```python
from build123d import *

# Parameters (mm, degrees)
SKETCH1_W                      = 247
SKETCH1_H                      = 127
BOSS_EXTRUDE1_DEPTH            = 63.5
M3X0_5_TAPPED_HOLE1_AT_2_COUNT = 2
M3X0_5_TAPPED_HOLE1_AT_2_PITCH = 20
M3X0_5_TAPPED_HOLE1_AT_3_COUNT = 2
M3X0_5_TAPPED_HOLE1_AT_3_PITCH = 220.907220344
M3X0_5_TAPPED_HOLE1_AT_4_COUNT = 2
M3X0_5_TAPPED_HOLE1_AT_4_PITCH = 220
SKETCH4_W                      = 19.05
SKETCH4_H                      = 6.35
BOSS_EXTRUDE2_DEPTH            = 5
SKETCH5_W                      = 1.5875
SKETCH5_H                      = 6.35
BOSS_EXTRUDE3_DEPTH            = 5


with BuildPart() as part:
    # Sketch1 → Boss-Extrude1 (new body)
    with BuildSketch(Plane(origin=(0, 0, 0), x_dir=(1, 0, 0), z_dir=(0, 1, 0))):
        Rectangle(SKETCH1_W, SKETCH1_H)
    extrude(amount=BOSS_EXTRUDE1_DEPTH)

    # Sketch3 → M3x0.5 Tapped Hole1 (revolve, cut)
    with BuildSketch(Plane(origin=(-112.5, 33.5, 63.5), x_dir=(0, -1, 0), z_dir=(1, 0, 0))):
        Polygon((0, 0), (0, 4.751075774), (1.25, 4), (1.25, 0), align=None)
    m3x0_5_tapped_hole1 = revolve(axis=Axis((-112.5, 33.5, 69.85), (0, 0, -1)), mode=Mode.SUBTRACT)

    # M3x0.5 Tapped Hole1 at 2: M3x0.5 Tapped Hole1 ×2
    with Locations(*[(0, -i * M3X0_5_TAPPED_HOLE1_AT_2_PITCH, 0) for i in range(1, M3X0_5_TAPPED_HOLE1_AT_2_COUNT)]):
        add(m3x0_5_tapped_hole1, mode=Mode.SUBTRACT)

    # M3x0.5 Tapped Hole1 at 3: M3x0.5 Tapped Hole1 ×2
    with Locations(*[Vector(0.9958932064677039, -0.09053574604251853, 0) * (i * M3X0_5_TAPPED_HOLE1_AT_3_PITCH) for i in range(1, M3X0_5_TAPPED_HOLE1_AT_3_COUNT)]):
        add(m3x0_5_tapped_hole1, mode=Mode.SUBTRACT)

    # M3x0.5 Tapped Hole1 at 4: M3x0.5 Tapped Hole1 ×2
    with Locations(*[(i * M3X0_5_TAPPED_HOLE1_AT_4_PITCH, 0, 0) for i in range(1, M3X0_5_TAPPED_HOLE1_AT_4_COUNT)]):
        add(m3x0_5_tapped_hole1, mode=Mode.SUBTRACT)

    # Mirror1: M3x0.5 Tapped Hole1 across plane
    add(m3x0_5_tapped_hole1.mirror(Plane.XY), mode=Mode.SUBTRACT)

    # Mirror1 copy 1 sketch → Mirror1 copy 1 (revolve, cut)
    with BuildSketch(Plane(origin=(-112.5, 13.5, -63.5), x_dir=(0, -1, 0), z_dir=(1, 0, 0))):
        Polygon((0, 0), (0, -4.751075774), (1.25, -4), (1.25, 0), align=None)
    revolve(axis=Axis((-112.5, 13.5, -69.85), (0, 0, -1)), mode=Mode.SUBTRACT)

    # Mirror1 copy 2 sketch → Mirror1 copy 2 (revolve, cut)
    with BuildSketch(Plane(origin=(107.5, 13.5, -63.5), x_dir=(0, -1, 0), z_dir=(1, 0, 0))):
        Polygon((0, 0), (0, -4.751075774), (1.25, -4), (1.25, 0), align=None)
    revolve(axis=Axis((107.5, 13.5, -69.85), (0, 0, -1)), mode=Mode.SUBTRACT)

    # Mirror1 copy 3 sketch → Mirror1 copy 3 (revolve, cut)
    with BuildSketch(Plane(origin=(107.5, 33.5, -63.5), x_dir=(0, -1, 0), z_dir=(1, 0, 0))):
        Polygon((0, 0), (0, -4.751075774), (1.25, -4), (1.25, 0), align=None)
    revolve(axis=Axis((107.5, 33.5, -69.85), (0, 0, -1)), mode=Mode.SUBTRACT)

    # Sketch4 → Boss-Extrude2 (add)
    with BuildSketch(Plane.ZY.offset(123.5)):
        with Locations((38.975, 15.175)):
            Rectangle(SKETCH4_W, SKETCH4_H)
    extrude(amount=BOSS_EXTRUDE2_DEPTH)

    # Sketch5 → Boss-Extrude3 (add)
    with BuildSketch(Plane.ZY.offset(128.5)):
        with Locations((30.24375, 15.175)):
            Rectangle(SKETCH5_W, SKETCH5_H)
        with Locations((36.064583333, 15.175)):
            Rectangle(SKETCH5_W, SKETCH5_H)
        with Locations((47.70625, 15.175)):
            Rectangle(SKETCH5_W, SKETCH5_H)
        with Locations((41.885416667, 15.175)):
            Rectangle(SKETCH5_W, SKETCH5_H)
    extrude(amount=BOSS_EXTRUDE3_DEPTH)


solid = part.part
```
Build history of the part. All positions in model axes, mm. A direction names the side the tool comes from. Coordinates: 2 decimals unless noted, no trailing zeros. Order: outer loops, then holes, each group sorted by start corner. A loop starts at its lowest first (then second) coordinate and runs counter-clockwise, first axis right, second up.
Item 1: Tool access for faces 4 (the flat face through (-127, 18.35, 39)), 5 (the flat face through (-127, 12, 39)), 6 (the flat face through (-131, 15, 42.679)): list every direction of +Z, -Z, +X, -X, +Y, -Y with a clear straight run to the whole face (end or side of a thin tool).
Filled in:
face 4: +Z, -Z, -X, +Y
face 5: +Z, -Z, -X, -Y
face 6: -X, +Y, -Y
Item 2: Saw through at A-A on y = 57.5. List the corners of the cut face in (x, z), then the cut area to 3 significant figures.
Filled in:
outline: (-123.5, -63.5) - (123.5, -63.5) - (123.5, 63.5) - (-123.5, 63.5) - close
area: 31,400 mm2
Item 3: Drill centre lines: L1, parallel to Y at x = -112.5, z = -61.25; L2, parallel to X at y = 33.5, z = 62.15; L3, parallel to X at y = 33, z = -60. Where is each one in solid material? Low to high.
Filled in:
L1: y = 0 to 12.25, 14.75 to 32.25, 34.75 to 63.5
L2: x = -123.5 to -113.75, -111.25 to 106.25, 108.75 to 123.5
L3: x = -123.5 to -113.65, -111.35 to 106.35, 108.65 to 123.5
Item 4: Mould opens along Z. For faces 1 (the flat face through (-131, 15, 35.271)), 2 (the flat face through (-128, 15, 29.45)), 3 (the flat face through (-2, 0, -1)) say: released by +Z, released by -Z, zero draft, split by the parting line, or undercut.
Filled in:
face 1: undercut
face 2: released by -Z
face 3: zero draft
Item 5: Saw through at B-B on z = -19.5. List the corners of the cut face in (x, y), then the cut area to 3 significant figures.
Filled in:
outline: (-123.5, 0) - (123.5, 0) - (123.5, 63.5) - (-123.5, 63.5) - close
area: 15,700 mm2
Item 6: Drop flat-ended pins along their axis: pin 1 Ø2 at (x, y) = (107.5, 33.5) entering from +Z; pin 2 Ø5 at (x, z) = (-127, 41.5) entering from -Y; pin 3 Ø3.5 at (y, z) = (17, 44.5) entering from -X. Give the stop position or say it passes through.
Filled in:
pin 1: stops at z = 59.35
pin 2: stops at y = 12
pin 3: stops at x = -128.5
